```python
from build123d import *

# Parameters (mm, degrees)
SKETCH1_W           = 25
SKETCH1_H           = 20
BOSS_EXTRUDE1_DEPTH = 4.5
SKETCH1_4_R         = 2.5
SKETCH1_4_R_2       = 1.4
CUT_EXTRUDE1_DEPTH  = 4.5


with BuildPart() as part:
    # Sketch1 → Boss-Extrude1 (new body)
    with BuildSketch(Plane(origin=(0, 0, 0), x_dir=(1, 0, 0), z_dir=(0, 1, 0))):
        with Locations((12.5, 10)):
            Rectangle(SKETCH1_W, SKETCH1_H)
    extrude(amount=BOSS_EXTRUDE1_DEPTH)

    # Sketch1<4> → Cut-Extrude1 (cut)
    with BuildSketch(Plane(origin=(0, 0, 0), x_dir=(1, 0, 0), z_dir=(0, 1, 0))):
        with Locations((5, 10)):
            Circle(SKETCH1_4_R)
        with Locations((20, 15)):
            Circle(SKETCH1_4_R_2)
        with Locations((20, 5)):
            Circle(SKETCH1_4_R_2)
    extrude(amount=CUT_EXTRUDE1_DEPTH, mode=Mode.SUBTRACT)


solid = part.part
```
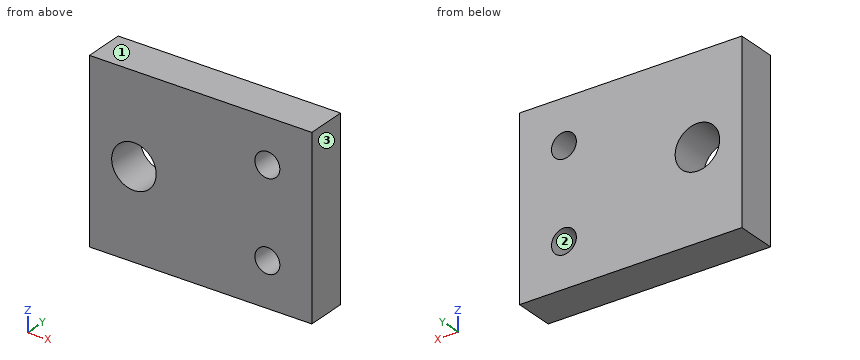
Part model, mm, in its own coordinate system. Face numbers are marked on the shaded views. Round coordinates to 2 decimals unless told otherwise and drop trailing zeros. Order: outer loops, then holes, each group sorted by start corner. A loop starts at its lowest first (then second) coordinate and runs counter-clockwise, first axis right, second up. Notation, with made-up numbers: M -35.75,70 L -2.75,70 A22 ccw -2.75,81 Z; hole C 42.25,-34 d9. An arc over 180 degrees is marked long. Answer in a Markdown table with one row per item. Add a question column.
Q1. Cut at A-A on x = 7. Give the cut face in (y, z), and give its area (3 significant figures).
Q2. Cut at C-C on z = -11.5. Give the cut face in (x, y).
Q3. Wall check: L1, parallel to Z at x = 20, y = 2.15; L2, parallel to X at y = 1.2, z = -10; L3, parallel to X at y = 0.85, z = -5. Give the ranges that are in metal, low to high. Write a range as from..to.
Q4. Cut at D-D on x = 20. Give the cut face in (y, z), and give its area (3 significant figures).
Q5. Mould opens along X. For the marked faces 1, 2 and 3 say: +X half, -X half, draft (parallel to the pull), parting line (faces both ways), or undercut.
Q6. Cut at B-B on y = 3.7. Give the cut face in (x, z).
Established:
| question | item | result |
|---|---|---|
| 1 | outline | M 0,-20 L 4.5,-20 L 4.5,-11.5 L 0,-11.5 Z; M 0,-8.5 L 4.5,-8.5 L 4.5,0 L 0,0 Z |
| 1 | area | 76.5 mm2 |
| 2 | outline | M 0,0 L 3,0 L 3,4.5 L 0,4.5 Z; M 7,0 L 25,0 L 25,4.5 L 7,4.5 Z |
| 3 | L1 | z = -20..-16.4, -13.6..-6.4, -3.6..0 |
| 3 | L2 | x = 0..2.5, 7.5..25 |
| 3 | L3 | x = 0..18.6, 21.4..25 |
| 4 | outline | M 0,-20 L 4.5,-20 L 4.5,-16.4 L 0,-16.4 Z; M 0,-13.6 L 4.5,-13.6 L 4.5,-6.4 L 0,-6.4 Z; M 0,-3.6 L 4.5,-3.6 L 4.5,0 L 0,0 Z |
| 4 | area | 64.8 mm2 |
| 5 | face 1 | draft |
| 5 | face 2 | undercut |
| 5 | face 3 | +X half |
| 6 | outline | M 0,-20 L 25,-20 L 25,0 L 0,0 Z; hole C 5,-10 d5; hole C 20,-15 d2.8; hole C 20,-5 d2.8 |
